```python
from build123d import *

# Parameters (mm, degrees)
SKETCH1_R                = 2
BOSS_EXTRUDE1_DEPTH      = 15
BOSS_EXTRUDE1_DEPTH_BACK = 15


with BuildPart() as part:
    # Sketch1 → Boss-Extrude1 (new body, two sides)
    with BuildSketch(Plane.XY) as boss_extrude1_sk:
        with BuildLine():
            Line((-34.940571089, 130.399986549), (-38.822856765, 144.888873943))
            ThreePointArc((-38.822856765, 144.888873943), (0, 150), (38.822856765, 144.888873943))
            Line((38.822856765, 144.888873943), (34.940571089, 130.399986549))
            ThreePointArc((34.940571089, 130.399986549), (0, 135), (-34.940571089, 130.399986549))
        make_face()
        with Locations((0, 142.5)):
            Circle(SKETCH1_R, mode=Mode.SUBTRACT)
    extrude(amount=BOSS_EXTRUDE1_DEPTH)
    extrude(boss_extrude1_sk.sketch, amount=-BOSS_EXTRUDE1_DEPTH_BACK)


solid = part.part
```
CAD build for the part. Positions are in the model's coordinates, mm. Round coordinates to 2 decimals unless told otherwise and drop trailing zeros. Loops run counter-clockwise (first coordinate to the right, second up) from the corner with the lowest first, then second, coordinate; pieces in that order, holes last. Notation, with made-up numbers: M 42.5,-35 L 94.5,-35 A31 ccw 94.5,-2 Z; hole C -17,76 d1. An arc over 180 degrees is marked long. Use a Markdown table: item, result. Add a question column.
(1) Flat gauge pins, fed straight in: pin 1 (5 mm diameter, centred on x = 17.5, z = 3.5, fed in from +Y); pin 2 (2 mm diameter, centred on x = -27.5, z = 4, fed in from +Y); pin 3 (8 mm diameter, centred on x = -3.5, z = -7.5, fed in from -Y); pin 4 (5 mm diameter, centred on x = 0, y = 142.5, fed in from -Z). Where does each tip first touch, or does it go through?
(2) Pull direction X, two halves, no side cores. Call faces 1 (the face through (0, 135, 0)), 2 (the face through (-36.855, 137.543, 0.21)), 3 (the face through (1, 140, -15)): +X half, -X half, draft (parallel to the pull), parting line (faces both ways), or undercut.
(3) Drill centre lines: line 1 (Y direction, x = 0, z = -6.75); line 2 (X direction, y = 142.5, z = 8); line 3 (X direction, y = 138.5, z = 6). Where is each one in solid material? Low to high.
(4) Cut at C-C (y = 142.5). Give the cut face in (x, z).
(5) Cut at B-B (z = 11). Give the cut face in (x, y), and give its area (3 significant figures).
(6) Cut at A-A (x = 0). Give the cut face in (y, z), and give its area (3 significant figures).
(7) Cut at D-D (x = 33). Give the cut face in (y, z).
Geometry says:
| question | item | result |
|---|---|---|
| 1 | pin 1 | stops at y = 149.25 |
| 1 | pin 2 | stops at y = 147.64 |
| 1 | pin 3 | stops at y = 134.79 |
| 1 | pin 4 | stops at z = -15 |
| 2 | face 1 | undercut |
| 2 | face 2 | -X half |
| 2 | face 3 | draft |
| 3 | line 1 | y = 135 to 140.5, 144.5 to 150 |
| 3 | line 2 | x = -38.18 to -2, 2 to 38.18 |
| 3 | line 3 | x = -37.11 to 37.11 |
| 4 | outline | M -38.18,-15 L -2,-15 L -2,15 L -38.18,15 Z; M 2,-15 L 38.18,-15 L 38.18,15 L 2,15 Z |
| 5 | outline | M -38.82,144.89 L -34.94,130.4 A135 cw 34.94,130.4 L 38.82,144.89 A150 ccw Z; hole C 0,142.5 d4 |
| 5 | area | 1,110 mm² |
| 6 | outline | M 135,-15 L 140.5,-15 L 140.5,15 L 135,15 Z; M 144.5,-15 L 150,-15 L 150,15 L 144.5,15 Z |
| 6 | area | 330 mm² |
| 7 | outline | M 130.9,-15 L 146.32,-15 L 146.32,15 L 130.9,15 Z |
